Can you work these out from the model? Positions are in its coordinate system, mm. Face numbers are marked on the shaded views. A direction names the side the tool comes from. Round coordinates to 2 decimals unless told otherwise and drop trailing zeros. Loops run counter-clockwise (first coordinate to the right, second up) from the corner with the lowest first, then second, coordinate; pieces in that order, holes last.
(1) I want a section at B-B on x = -23.5. Write out the boundary of the cut face in (y, z).
(2) Will these pins go through, and if not, where does the flat tip stop? pin 1 Ø2 at (x, z) = (91.06, 9) entering from -Y; pin 2 Ø1.6 at (y, z) = (44.5, 62.5) entering from +X; pin 3 Ø1.6 at (x, y) = (16.5, -1) entering from -Z; pin 4 Ø0.6 at (y, z) = (-1.5, 71.5) entering from -X.
(3) Which directions (+Z, -Z, +X, -X, +Y, -Y) give clear straight access to the entire face, cutting with the end or side of a thin tool? Please do the marked faces 4 and 5.
(4) If I drill on line 1 along Z through (x, y) = (-72.45, 10.6); line 2 along Y through (x, z) = (81, 101.5); line 3 along X through (y, z) = (36, 103.5), over which ranges is the centre line in solid material (lowest first)?
(5) I want a section at C-C on z = 100.5. Write out the boundary of the cut face in (x, y).
(6) Thinking about a two-plate mould opening in Y: for the marked faces 1, 2 and 3, which applies, released by +Y, released by -Y, zero draft, split by the parting line, or undercut?
(7) I want a section at D-D on z = 47. Give the number of separate pieces and of enclosed holes in the cut face, plus the area to 3 significant figures.
(8) I want a section at A-A on y = 28. Write out the boundary of the cut face in (x, z).
from build123d import *

# Parameters (mm, degrees)
ESBO_O1_W                 = 174
ESBO_O1_H                 = 2
EXTRUS_O_FINA1_DEPTH      = 124
ESBO_O2_R                 = 1.25
CORTE_EXTRUS_O1_DEPTH     = 10
ESBO_O3_W                 = 2
ESBO_O3_H                 = 124
RESSALTO_EXTRUS_O1_DEPTH  = 45.2
ESBO_O4_W                 = 124
ESBO_O4_H                 = 2
RESSALTO_EXTRUS_O2_DEPTH  = 34
ESBO_O5_W                 = 124
ESBO_O5_H                 = 2
RESSALTO_EXTRUS_O3_DEPTH  = 34
CORTE_EXTRUS_O2_REACH     = 220.392
ESBO_O6_R                 = 1.35
ESBO_O6_W                 = 59.5
ESBO_O6_H                 = 29
ESBO_O7_R                 = 1.5
CORTE_EXTRUS_O3_DEPTH     = 2
ESBO_O8_W                 = 22.175
ESBO_O8_H                 = 48
CORTE_EXTRUS_O4_DEPTH     = 2
CONVERTER_S_LIDO1_DEPTH   = 124
CONVERTER_S_LIDO1_2_DEPTH = 124


# Read off the part's stored shape, not the designer's step: Converter-Sólido1
with BuildPart() as part:
    # Esboço1 → Extrusão-Fina1 (new body)
    with BuildSketch(Plane.XY):
        with Locations((13.061802497, -1)):
            Rectangle(ESBO_O1_W, ESBO_O1_H)
    extrude(amount=EXTRUS_O_FINA1_DEPTH)

    # Esboço2 → Corte-extrusão1 (cut)
    with BuildSketch(Plane(origin=(0, 0, 0), x_dir=(1, 0, 0), z_dir=(0, 1, 0))):
        with Locations(Location((-64.938197503, -9, 0), (0, 0, 270))):
            Circle(ESBO_O2_R)
        with Locations(Location((-64.938197503, -115, 0), (0, 0, 270))):
            Circle(ESBO_O2_R)
        with Locations(Location((91.061802497, -115, 0), (0, 0, 270))):
            Circle(ESBO_O2_R)
        with Locations(Location((91.061802497, -9, 0), (0, 0, 270))):
            Circle(ESBO_O2_R)
    extrude(amount=-CORTE_EXTRUS_O1_DEPTH, mode=Mode.SUBTRACT)

    # Esboço3 → Ressalto-extrusão1 (add)
    with BuildSketch(Plane(origin=(0, 0, 0), x_dir=(1, 0, 0), z_dir=(0, 1, 0))):
        with Locations((-72.938197503, -62)):
            Rectangle(ESBO_O3_W, ESBO_O3_H)
        with Locations((99.061802497, -62)):
            Rectangle(ESBO_O3_W, ESBO_O3_H)
    extrude(amount=RESSALTO_EXTRUS_O1_DEPTH)

    # Esboço4 → Ressalto-extrusão2 (add)
    with BuildSketch(Plane(origin=(-71.938197503, 0, 0), x_dir=(0, 0, -1), z_dir=(1, 0, 0))):
        with Locations((-62, 44.2)):
            Rectangle(ESBO_O4_W, ESBO_O4_H)
    extrude(amount=RESSALTO_EXTRUS_O2_DEPTH)

    # Esboço5 → Ressalto-extrusão3 (add)
    with BuildSketch(Plane.ZY.offset(-98.061802497)):
        with Locations((62, 44.2)):
            Rectangle(ESBO_O5_W, ESBO_O5_H)
    extrude(amount=RESSALTO_EXTRUS_O3_DEPTH)

    # Esboço6 → Corte-extrusão2 (cut, up to next)
    with BuildSketch(Plane(origin=(100.061802497, 0, 0), x_dir=(0, 0, -1), z_dir=(1, 0, 0)), mode=Mode.PRIVATE) as corte_extrus_o2_sk1:
        with Locations(Location((-86.75, 38.9, 0), (0, 0, 180))):
            Circle(ESBO_O6_R)
    corte_extrus_o2_tool1 = extrude(corte_extrus_o2_sk1.sketch, amount=-CORTE_EXTRUS_O2_REACH, mode=Mode.PRIVATE) & part.part
    # Esboço6 → Corte-extrusão2 (cut, up to next)
    with BuildSketch(Plane(origin=(100.061802497, 0, 0), x_dir=(0, 0, -1), z_dir=(1, 0, 0)), mode=Mode.PRIVATE) as corte_extrus_o2_sk2:
        with Locations(Location((-64.75, 38.9, 0), (0, 0, 180))):
            Circle(ESBO_O6_R)
    corte_extrus_o2_tool2 = extrude(corte_extrus_o2_sk2.sketch, amount=-CORTE_EXTRUS_O2_REACH, mode=Mode.PRIVATE) & part.part
    # Esboço6 → Corte-extrusão2 (cut, up to next)
    with BuildSketch(Plane(origin=(100.061802497, 0, 0), x_dir=(0, 0, -1), z_dir=(1, 0, 0)), mode=Mode.PRIVATE) as corte_extrus_o2_sk3:
        with Locations(Location((-42.75, 38.9, 0), (0, 0, 180))):
            Circle(ESBO_O6_R)
    corte_extrus_o2_tool3 = extrude(corte_extrus_o2_sk3.sketch, amount=-CORTE_EXTRUS_O2_REACH, mode=Mode.PRIVATE) & part.part
    # Esboço6 → Corte-extrusão2 (cut, up to next)
    with BuildSketch(Plane(origin=(100.061802497, 0, 0), x_dir=(0, 0, -1), z_dir=(1, 0, 0)), mode=Mode.PRIVATE) as corte_extrus_o2_sk4:
        with Locations(Location((-86.75, 4.3, 0), (0, 0, 180))):
            Circle(ESBO_O6_R)
    corte_extrus_o2_tool4 = extrude(corte_extrus_o2_sk4.sketch, amount=-CORTE_EXTRUS_O2_REACH, mode=Mode.PRIVATE) & part.part
    # Esboço6 → Corte-extrusão2 (cut, up to next)
    with BuildSketch(Plane(origin=(100.061802497, 0, 0), x_dir=(0, 0, -1), z_dir=(1, 0, 0)), mode=Mode.PRIVATE) as corte_extrus_o2_sk5:
        with Locations(Location((-64.75, 4.3, 0), (0, 0, 180))):
            Circle(ESBO_O6_R)
    corte_extrus_o2_tool5 = extrude(corte_extrus_o2_sk5.sketch, amount=-CORTE_EXTRUS_O2_REACH, mode=Mode.PRIVATE) & part.part
    # Esboço6 → Corte-extrusão2 (cut, up to next)
    with BuildSketch(Plane(origin=(100.061802497, 0, 0), x_dir=(0, 0, -1), z_dir=(1, 0, 0)), mode=Mode.PRIVATE) as corte_extrus_o2_sk6:
        with Locations(Location((-42.75, 4.3, 0), (0, 0, 180))):
            Circle(ESBO_O6_R)
    corte_extrus_o2_tool6 = extrude(corte_extrus_o2_sk6.sketch, amount=-CORTE_EXTRUS_O2_REACH, mode=Mode.PRIVATE) & part.part
    # Esboço6 → Corte-extrusão2 (cut, up to next)
    with BuildSketch(Plane(origin=(100.061802497, 0, 0), x_dir=(0, 0, -1), z_dir=(1, 0, 0)), mode=Mode.PRIVATE) as corte_extrus_o2_sk7:
        with Locations(Location((-94.55, 32.6, 0), (0, 0, 180))):
            Circle(ESBO_O6_R)
    corte_extrus_o2_tool7 = extrude(corte_extrus_o2_sk7.sketch, amount=-CORTE_EXTRUS_O2_REACH, mode=Mode.PRIVATE) & part.part
    # Esboço6 → Corte-extrusão2 (cut, up to next)
    with BuildSketch(Plane(origin=(100.061802497, 0, 0), x_dir=(0, 0, -1), z_dir=(1, 0, 0)), mode=Mode.PRIVATE) as corte_extrus_o2_sk8:
        with Locations(Location((-94.55, 10.6, 0), (0, 0, 180))):
            Circle(ESBO_O6_R)
    corte_extrus_o2_tool8 = extrude(corte_extrus_o2_sk8.sketch, amount=-CORTE_EXTRUS_O2_REACH, mode=Mode.PRIVATE) & part.part
    # Esboço6 → Corte-extrusão2 (cut, up to next)
    with BuildSketch(Plane(origin=(100.061802497, 0, 0), x_dir=(0, 0, -1), z_dir=(1, 0, 0)), mode=Mode.PRIVATE) as corte_extrus_o2_sk9:
        with Locations((-62, 21.6)):
            Rectangle(ESBO_O6_W, ESBO_O6_H)
    corte_extrus_o2_tool9 = extrude(corte_extrus_o2_sk9.sketch, amount=-CORTE_EXTRUS_O2_REACH, mode=Mode.PRIVATE) & part.part
    add(corte_extrus_o2_tool1.solids().sort_by_distance((100.061802, 38.9, 86.75))[0], mode=Mode.SUBTRACT)
    add(corte_extrus_o2_tool1.solids().sort_by_distance((100.061802, 38.9, 86.75))[1], mode=Mode.SUBTRACT)
    add(corte_extrus_o2_tool2.solids().sort_by_distance((100.061802, 38.9, 64.75))[0], mode=Mode.SUBTRACT)
    add(corte_extrus_o2_tool2.solids().sort_by_distance((100.061802, 38.9, 64.75))[1], mode=Mode.SUBTRACT)
    add(corte_extrus_o2_tool3.solids().sort_by_distance((100.061802, 38.9, 42.75))[0], mode=Mode.SUBTRACT)
    add(corte_extrus_o2_tool3.solids().sort_by_distance((100.061802, 38.9, 42.75))[1], mode=Mode.SUBTRACT)
    add(corte_extrus_o2_tool4.solids().sort_by_distance((100.061802, 4.3, 86.75))[0], mode=Mode.SUBTRACT)
    add(corte_extrus_o2_tool4.solids().sort_by_distance((100.061802, 4.3, 86.75))[1], mode=Mode.SUBTRACT)
    add(corte_extrus_o2_tool5.solids().sort_by_distance((100.061802, 4.3, 64.75))[0], mode=Mode.SUBTRACT)
    add(corte_extrus_o2_tool5.solids().sort_by_distance((100.061802, 4.3, 64.75))[1], mode=Mode.SUBTRACT)
    add(corte_extrus_o2_tool6.solids().sort_by_distance((100.061802, 4.3, 42.75))[0], mode=Mode.SUBTRACT)
    add(corte_extrus_o2_tool6.solids().sort_by_distance((100.061802, 4.3, 42.75))[1], mode=Mode.SUBTRACT)
    add(corte_extrus_o2_tool7.solids().sort_by_distance((100.061802, 32.6, 94.55))[0], mode=Mode.SUBTRACT)
    add(corte_extrus_o2_tool7.solids().sort_by_distance((100.061802, 32.6, 94.55))[1], mode=Mode.SUBTRACT)
    add(corte_extrus_o2_tool8.solids().sort_by_distance((100.061802, 10.6, 94.55))[0], mode=Mode.SUBTRACT)
    add(corte_extrus_o2_tool8.solids().sort_by_distance((100.061802, 10.6, 94.55))[1], mode=Mode.SUBTRACT)
    add(corte_extrus_o2_tool9.solids().sort_by_distance((100.061802, 21.6, 62))[0], mode=Mode.SUBTRACT)
    add(corte_extrus_o2_tool9.solids().sort_by_distance((100.061802, 21.6, 62))[1], mode=Mode.SUBTRACT)

    # Esboço7 → Corte-extrusão3 (cut)
    with BuildSketch(Plane(origin=(0, 45.2, 0), x_dir=(1, 0, 0), z_dir=(0, 1, 0))):
        with Locations(Location((-63.938197503, -10, 0), (0, 0, 270))):
            Circle(ESBO_O7_R)
        with Locations(Location((90.061802497, -10, 0), (0, 0, 270))):
            Circle(ESBO_O7_R)
        with Locations(Location((90.061802497, -114, 0), (0, 0, 270))):
            Circle(ESBO_O7_R)
        with Locations(Location((-63.938197503, -114, 0), (0, 0, 270))):
            Circle(ESBO_O7_R)
    extrude(amount=-CORTE_EXTRUS_O3_DEPTH, mode=Mode.SUBTRACT)

    # Esboço8 → Corte-extrusão4 (cut)
    with BuildSketch(Plane(origin=(0, 0, 0), x_dir=(1, 0, 0), z_dir=(0, 1, 0))):
        with Locations((-25.155697503, -61.66)):
            Rectangle(ESBO_O8_W, ESBO_O8_H)
        with BuildLine():
            Line((90.106802497, -34.3), (90.106802497, -82.3))
            ThreePointArc((90.106802497, -82.3), (82.606802497, -89.8), (75.106802497, -82.3))
            Line((75.106802497, -82.3), (75.106802497, -34.3))
            ThreePointArc((75.106802497, -34.3), (82.606802497, -26.8), (90.106802497, -34.3))
        make_face()
        with Locations((17.019302497, -61.66)):
            Rectangle(ESBO_O8_W, ESBO_O8_H)
        with BuildLine():
            Line((66.606802497, -34.3), (66.606802497, -82.3))
            ThreePointArc((66.606802497, -82.3), (59.106802497, -89.8), (51.606802497, -82.3))
            Line((51.606802497, -82.3), (51.606802497, -34.3))
            ThreePointArc((51.606802497, -34.3), (59.106802497, -26.8), (66.606802497, -34.3))
        make_face()
    extrude(amount=-CORTE_EXTRUS_O4_DEPTH, mode=Mode.SUBTRACT)

    # Converter-Sólido1 outline → Converter-Sólido1 (cut)
    with BuildSketch(Plane.XY):
        with BuildLine():
            ThreePointArc((96.061802497, 45.2), (98.890229621, 44.028427124), (100.061802497, 41.2))
            Line((100.061802497, 41.2), (100.061802497, 45.2))
            Line((100.061802497, 45.2), (96.061802497, 45.2))
        make_face()
        with BuildLine():
            ThreePointArc((100.061802497, 2), (98.890229621, -0.828427125), (96.061802497, -2))
            Line((96.061802497, -2), (100.061802497, -2))
            Line((100.061802497, -2), (100.061802497, 2))
        make_face()
        with BuildLine():
            ThreePointArc((-69.938197503, -2), (-72.766624628, -0.828427125), (-73.938197503, 2))
            Line((-73.938197503, 2), (-73.938197503, -2))
            Line((-73.938197503, -2), (-69.938197503, -2))
        make_face()
        with BuildLine():
            ThreePointArc((-73.938197503, 41.2), (-72.766624628, 44.028427125), (-69.938197503, 45.2))
            Line((-69.938197503, 45.2), (-73.938197503, 45.2))
            Line((-73.938197503, 45.2), (-73.938197503, 41.2))
        make_face()
    extrude(amount=CONVERTER_S_LIDO1_DEPTH, mode=Mode.SUBTRACT)

    # Converter-S_lido1 2 outline → Converter-S_lido1 2 (add)
    with BuildSketch(Plane.XY):
        with BuildLine():
            ThreePointArc((96.061802497, 43.2), (97.476016059, 42.614213562), (98.061802497, 41.2))
            Line((98.061802497, 41.2), (98.061802497, 43.2))
            Line((98.061802497, 43.2), (96.061802497, 43.2))
        make_face()
        with BuildLine():
            ThreePointArc((98.061802497, 2), (97.476016059, 0.585786438), (96.061802497, 0))
            Line((96.061802497, 0), (98.061802497, 0))
            Line((98.061802497, 0), (98.061802497, 2))
        make_face()
        with BuildLine():
            ThreePointArc((-69.938197503, 0), (-71.352411066, 0.585786437), (-71.938197503, 2))
            Line((-71.938197503, 2), (-71.938197503, 0))
            Line((-71.938197503, 0), (-69.938197503, 0))
        make_face()
        with BuildLine():
            ThreePointArc((-71.938197503, 41.2), (-71.352411066, 42.614213563), (-69.938197503, 43.2))
            Line((-69.938197503, 43.2), (-71.938197503, 43.2))
            Line((-71.938197503, 43.2), (-71.938197503, 41.2))
        make_face()
    extrude(amount=CONVERTER_S_LIDO1_2_DEPTH)


solid = part.part
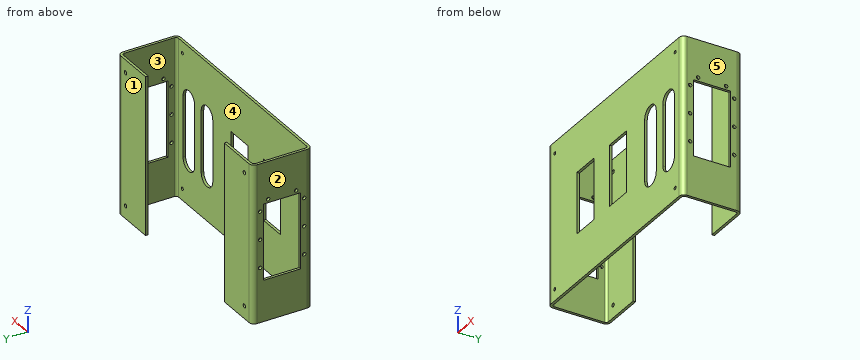
Filled sheet:
1. outline: (-2, 0) - (0, 0) - (0, 37.66) - (-2, 37.66) - close; (-2, 85.66) - (0, 85.66) - (0, 124) - (-2, 124) - close
2. pin 1: stops at y = 43.2
2. pin 2: stops at x = 99.18
2. pin 3: stops at z = 0
2. pin 4: stops at x = -72.34
3. face 4: +Z, -Z
3. face 5: +Z, -Z, +X, +Y, -Y
4. line 1: z = 0 to 32.25, 91.75 to 93.2, 95.9 to 124
4. line 2: y = -2 to 0, 43.2 to 45.2
4. line 3: x = -73.94 to -71.94, 98.06 to 100.06
5. outline: (-73.94, 2) arc R4 ccw to (-69.94, -2) - (96.06, -2) arc R4 ccw to (100.06, 2) - (100.06, 41.2) arc R4 ccw to (96.06, 45.2) - (64.06, 45.2) - (64.06, 43.2) - (96.06, 43.2) arc R2 cw to (98.06, 41.2) - (98.06, 2) arc R2 cw to (96.06, 0) - (-69.94, 0) arc R2 cw to (-71.94, 2) - (-71.94, 41.2) arc R2 cw to (-69.94, 43.2) - (-37.94, 43.2) - (-37.94, 45.2) - (-69.94, 45.2) arc R4 ccw to (-73.94, 41.2) - close
6. face 1: released by +Y
6. face 2: zero draft
6. face 3: undercut
7. separate pieces: 7
7. enclosed holes: 0
7. area: 390 mm2
8. outline: (-73.94, 0) - (-71.94, 0) - (-71.94, 32.25) - (-73.94, 32.25) - close; (-73.94, 91.75) - (-71.94, 91.75) - (-71.94, 124) - (-73.94, 124) - close; (98.06, 0) - (100.06, 0) - (100.06, 32.25) - (98.06, 32.25) - close; (98.06, 91.75) - (100.06, 91.75) - (100.06, 124) - (98.06, 124) - close
